Design review of the part built by this model. Coordinates are the model's own, in mm. A direction names the side the tool comes from. Give positions to 0.01 mm unless a question says otherwise; leave off trailing zeros. Write each loop counter-clockwise with the first axis right and the second up, starting at its lowest first coordinate (ties: lowest second). Pieces come first, ordered by that corner, then holes.
```python
from build123d import *

# Parameters (mm, degrees)
ESQUISSE1_R                         = 8
BOSS_EXTRU_1_DEPTH                  = 20.8
DIAM_TRE_DU_PER_AGE_12_0_12_1_D     = 12
DIAM_TRE_DU_PER_AGE_12_0_12_1_DEPTH = 88
DIAM_TRE_DU_PER_AGE_12_0_12_1_TIP   = 3.605163714
CONG_1_R                            = 7
ENL_V_MAT_EXTRU_1_DEPTH             = 109.892791429
ESQUISSE6_R                         = 3.25
ENL_V_MAT_EXTRU_2_DEPTH             = 10
TROU_TARAUD_M41_D                   = 3.3


with BuildPart() as part:
    # Esquisse1 → Boss.-Extru.1 (new, symmetric)
    with BuildSketch(Plane.XY):
        with BuildLine():
            Line((0, -10), (105, -10))
            Line((105, -10), (105, 10))
            Line((105, 10), (0, 10))
            ThreePointArc((0, 10), (-10, 0), (0, -10))
        make_face()
        Circle(ESQUISSE1_R, mode=Mode.SUBTRACT)
    extrude(amount=BOSS_EXTRU_1_DEPTH, both=True)

    # Diamètre du perçage Ø12.0 (12)1
    with Locations(Plane(origin=(105, 0, 0), x_dir=(0, 0, -1), z_dir=(1, 0, 0))):
        with Locations((0, 0)):
            Hole(DIAM_TRE_DU_PER_AGE_12_0_12_1_D / 2, depth=DIAM_TRE_DU_PER_AGE_12_0_12_1_DEPTH)
            with Locations((0, 0, -(DIAM_TRE_DU_PER_AGE_12_0_12_1_DEPTH + DIAM_TRE_DU_PER_AGE_12_0_12_1_TIP / 2))):  # 118° drill point
                Cone(0, DIAM_TRE_DU_PER_AGE_12_0_12_1_D / 2, DIAM_TRE_DU_PER_AGE_12_0_12_1_TIP, mode=Mode.SUBTRACT)

    # Congé1
    # the kernel refuses this fillet: 7 mm, written as the material it takes off along each edge
    with BuildSketch(Plane(origin=(105, 10, -38.3), x_dir=(0, -1, 0), z_dir=(0, 0, 1))) as cong_1_piece_1:
        with BuildLine():
            CenterArc((CONG_1_R, -CONG_1_R), CONG_1_R, 90, 90)
            Line((0, -CONG_1_R), (0, 0))
            Line((0, 0), (CONG_1_R, 0))
        make_face()
    extrude(amount=76.6, mode=Mode.SUBTRACT)

    # Esquisse5 → Enlèv. mat.-Extru.1 (cut, through all)
    with BuildSketch(Plane(origin=(0, 10, 0), x_dir=(1, 0, 0), z_dir=(0, 1, 0))):
        with BuildLine():
            Line((12, -12.5), (12, 12.5))
            ThreePointArc((12, 12.5), (12.585786438, 13.914213562), (14, 14.5))
            Line((14, 14.5), (14, 17))
            Line((14, 17), (17, 17))
            Line((17, 17), (17, 12.5))
            Line((17, 12.5), (23, 12.5))
            Line((23, 12.5), (23, -12.5))
            Line((23, -12.5), (17, -12.5))
            Line((17, -12.5), (17, -17))
            Line((17, -17), (14, -17))
            Line((14, -17), (14, -14.5))
            ThreePointArc((14, -14.5), (12.585786438, -13.914213562), (12, -12.5))
        make_face()
    extrude(amount=-ENL_V_MAT_EXTRU_1_DEPTH, mode=Mode.SUBTRACT)

    # Esquisse6 → Enlèv. mat.-Extru.2 (cut)
    with BuildSketch(Plane(origin=(0, 10, 0), x_dir=(1, 0, 0), z_dir=(0, 1, 0))):
        with Locations((23, 0)):
            Circle(ESQUISSE6_R)
    extrude(amount=-ENL_V_MAT_EXTRU_2_DEPTH, mode=Mode.SUBTRACT)

    # Trou taraudé M41 (through all)
    with Locations(Plane(origin=(0, 0, -20.8), x_dir=(-1, 0, 0), z_dir=(0, 0, -1))):
        with Locations((-15.5, 0)):
            Hole(TROU_TARAUD_M41_D / 2)


solid = part.part
```
(1) Clearance check with flat-ended pins moving along their axes: P1, Ø3, axis at y = 7.5, z = 15.5, coming from the +X side; P2, Ø5, axis at y = -5.5, z = -15.5, coming from the -X side; P3, Ø5, axis at y = -5, z = 15.5, coming from the -X side. State where each tip first meets the part, or that it passes through.
Resolved:
P1: stops at x = 104.32
P2: stops at x = -9.54
P3: stops at x = -9.68
(2) To check wall thickness, follow L1, parallel to X at y = 0.25, z = -7; L2, parallel to X at y = -7.25, z = 10; L3, parallel to Z at x = 86, y = 0.5. State the ranges of each line that lie inside material, in increasing order.
Resolved:
L1: x = -10 to -8, 8 to 12, 23 to 105
L2: x = -6.89 to -3.38, 3.38 to 12, 23 to 105
L3: z = -20.8 to -5.98, 5.98 to 20.8
(3) Consider section B-B, the plane z = -7. Give the boundary of the cut face in (x, y).
Resolved:
outline: (0, -10) - (12, -10) - (12, 10) - (0, 10) arc R10 ccw to start; (23, -10) - (105, -10) - (105, 3) arc R7 ccw to (98, 10) - (23, 10) - close; hole circle Ø16 at (0, 0)
(4) Consider section D-D, the plane x = 83. Give the boundary of the cut face in (y, z), then the cut area to 3 significant figures.
Resolved:
outline: (-10, -20.8) - (10, -20.8) - (10, 20.8) - (-10, 20.8) - close; hole circle Ø12 at (0, 0)
area: 719 mm2
(5) Mouldability with a two-part tool opening along Z and no side actions: class faces 1 (the face through (47, 0, -20.8)), 2 (the face through (17.074, 0.496, 17.63)), 3 (the face through (14, -5, 16)) as pulls with the +Z half, pulls with the -Z half, needs draft (parallel to the pull), parting line crosses it, or undercut.
Resolved:
face 1: pulls with the -Z half
face 2: needs draft
face 3: undercut
(6) Consider section A-A, the plane x = 15.5. Give the boundary of the cut face in (y, z), then the cut area to 3 significant figures.
Resolved:
outline: (-10, -20.8) - (-1.65, -20.8) - (-1.65, -17) - (-10, -17) - close; (-10, 17) - (-1.65, 17) - (-1.65, 20.8) - (-10, 20.8) - close; (1.65, -20.8) - (10, -20.8) - (10, -17) - (1.65, -17) - close; (1.65, 17) - (10, 17) - (10, 20.8) - (1.65, 20.8) - close
area: 127 mm2
(7) Consider section C-C, the plane z = 2. Give the boundary of the cut face in (x, y).
Resolved:
outline: (0, -10) - (12, -10) - (12, 10) - (0, 10) arc R10 ccw to start; (23, -10) - (105, -10) - (105, -5.66) - (23, -5.66) - close; (25.56, 5.66) - (104.48, 5.66) arc R7 ccw to (98, 10) - (25.56, 10) - close; hole circle Ø16 at (0, 0)
(8) Tool access review of faces 4 (the face through (17, -5, -15)), 5 (the face through (103, 7.9, -0.3)), 6 (the face through (26.25, 7.56, 0.07)): name each direction out of +Z, -Z, +X, -X, +Y, -Y from which nothing blocks a thin tool from reaching the whole face with its end or side.
Resolved:
face 4: +Y, -Y
face 5: +Z, -Z, +X, +Y
face 6: +Y
